Source: three-view drawing plus pictorial views. Frame: mm from the lowest corner of the part. A direction names the side the tool comes from. Give positions to 0.01 mm unless a question says otherwise; leave off trailing zeros. Order: outer loops, then holes, each group sorted by start corner. A loop starts at its lowest first (then second) coordinate and runs counter-clockwise, first axis right, second up. Notation, with made-up numbers: (42, 27.25) -> (61, 27.25) arc R29 cw to (61, 49.25) -> close; hole circle Ø9 at (74.5, -3). An arc over 180 degrees is marked (long way). Answer in a Markdown table with one row per item.
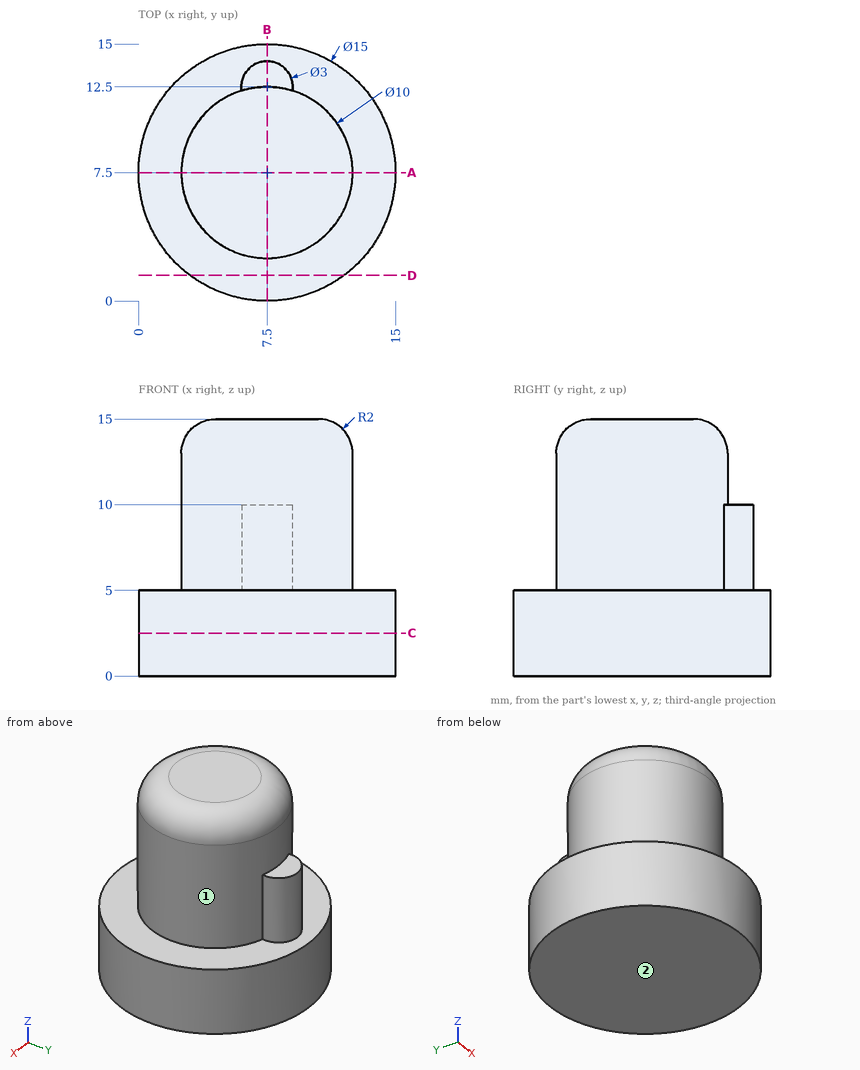
(1) Section query C-C (z = 2.5). Return the cut outline in (x, y).
A:
| item | result |
|---|---|
| outline | circle Ø15 at (7.5, 7.5) |
(2) First-contact query: pin 1 Ø1.9 at (x, y) = (8, 13.5) entering from +Z; pin 2 Ø2 at (x, y) = (11, 5) entering from +Z. Flat tips, straight axial feed; report the tip coordinate or a pass-through.
A:
| item | result |
|---|---|
| pin 1 | stops at z = 10 |
| pin 2 | stops at z = 14.98 |
(3) Section query A-A (y = 7.5). Return the cut outline in (x, z), plus the area to 3 significant figures.
A:
| item | result |
|---|---|
| outline | (0, 0) -> (15, 0) -> (15, 5) -> (12.5, 5) -> (12.5, 13) arc R2 ccw to (10.5, 15) -> (4.5, 15) arc R2 ccw to (2.5, 13) -> (2.5, 5) -> (0, 5) -> close |
| area | 173 mm^2 |
(4) Ray query, probe 1 along Z at (x, y) = (13, 6.5); probe 2 along Z at (x, y) = (8.75, 13); probe 3 along Y at (x, z) = (10.25, 2). Return the intervals inside material, ascending.
A:
| item | result |
|---|---|
| probe 1 | z = 0 to 5 |
| probe 2 | z = 0 to 10 |
| probe 3 | y = 0.52 to 14.48 |
(5) Access query for the marked faces 1 and 2. Directions: +Z, -Z, +X, -X, +Y, -Y. A direction counts if a zero-diameter tool reaches every point of the face in a straight line with its end or side. Return the directions, or none.
A:
| item | result |
|---|---|
| face 1 | +Z |
| face 2 | -Z, +X, -X, +Y, -Y |
(6) Section query B-B (x = 7.5). Return the cut outline in (y, z), plus the area to 3 significant figures.
A:
| item | result |
|---|---|
| outline | (0, 0) -> (15, 0) -> (15, 5) -> (14, 5) -> (14, 10) -> (12.5, 10) -> (12.5, 13) arc R2 ccw to (10.5, 15) -> (4.5, 15) arc R2 ccw to (2.5, 13) -> (2.5, 5) -> (0, 5) -> close |
| area | 181 mm^2 |
(7) Section query D-D (y = 1.5). Return the cut outline in (x, z).
A:
| item | result |
|---|---|
| outline | (3, 0) -> (12, 0) -> (12, 5) -> (3, 5) -> close |
